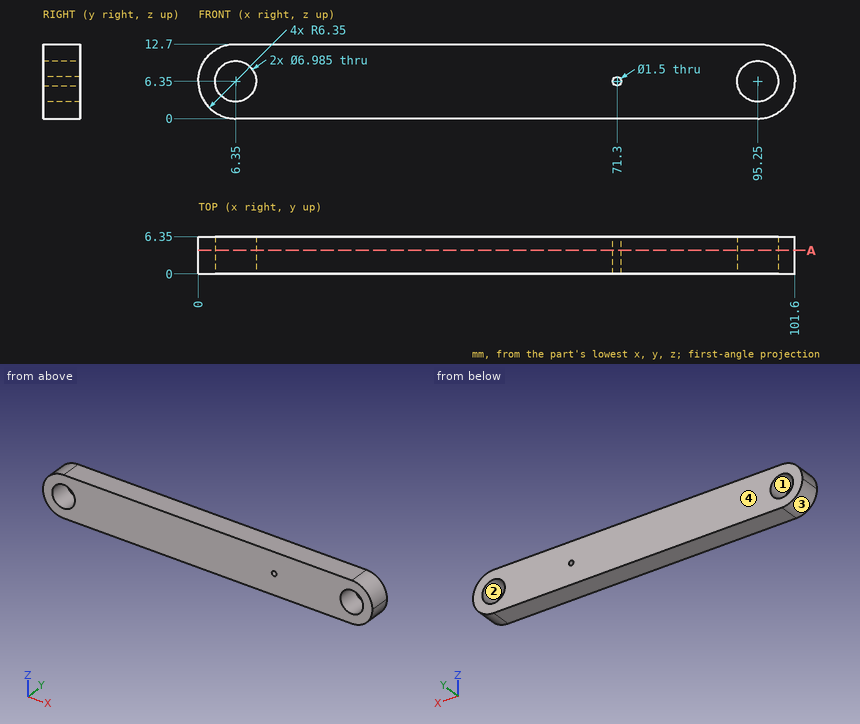
Part print with two shaded views. Sizes in mm from the minimum x, y, z corner. Coordinates: 2 decimals unless noted, no trailing zeros.
1. Drill centre lines: probe 1 along X at (y, z) = (5, 6.35); probe 2 along X at (y, z) = (5.75, 8.5) (1 decimal); probe 3 along X at (y, z) = (1.75, 6.75). Where is each one in solid material? Low to high.
Answer block:
probe 1: x = 0 to 2.86, 9.84 to 70.55, 72.05 to 91.76, 98.74 to 101.6
probe 2: x = 0.4 to 3.6, 9.1 to 92.5, 98 to 101.2
probe 3: x = 0.01 to 2.88, 9.82 to 70.67, 71.93 to 91.78, 98.72 to 101.59
2. Pull direction X, two halves, no side cores. Call the marked faces 1, 2, 3 and 4: released by +X, released by -X, zero draft, split by the parting line, or undercut.
Answer block:
face 1: undercut
face 2: undercut
face 3: released by -X
face 4: zero draft
3. Drop a flat-ended pin along its axis: pin 1 (1 mm diameter, centred on y = 5.5, z = 7.5, fed in from -X). Give the stop position or say it passes through.
Answer block:
pin 1: stops at x = 0.03
4. Band-saw the part on A-A, the plane y = 4. Give the number of separate pieces and of enclosed holes in the cut face, and give its area (3 significant figures).
Answer block:
separate pieces: 1
enclosed holes: 3
area: 1,180 mm2
